from build123d import *

# Parameters (mm, degrees)
F0_W     = 81.2149718404
F0_H     = 45.3068669885
F1_DEPTH = 50.8
F2_R     = 7.5673646555
F2_R_2   = 8.1937983632
F3_DEPTH = 25.4
F5_DEPTH = 25.4
F7_DEPTH = 25.4


with BuildPart() as f1:
    # F0 (on Top) → F1 (new body)
    with BuildSketch(Plane.XY):
        with Locations((15.9056037664, 3.0124252662)):
            Rectangle(F0_W, F0_H)
    extrude(amount=F1_DEPTH)

    # F2 (on face) → F3 (cut)
    with BuildSketch(Plane.XY.offset(50.8)):
        with Locations((-12.4111901969, 4.940376617)):
            Circle(F2_R)
        with Locations((42.7764281631, 4.4583887793)):
            Circle(F2_R_2)
    extrude(amount=-F3_DEPTH, mode=Mode.SUBTRACT)

    # F4 (on face) → F5 (cut)
    with BuildSketch(Plane.XZ.offset(19.6410082281)):
        with BuildLine():
            Line((34.1006480157, 50.8), (0, 50.8))
            ThreePointArc((0, 50.8), (17.0503240079, 39.4000553567), (34.1006480157, 50.8))
        make_face()
    extrude(amount=-F5_DEPTH, mode=Mode.SUBTRACT)

    # F6 (on face) → F7 (cut)
    with BuildSketch(Plane.XZ.offset(-5.7589917719)):
        with BuildLine():
            Line((34.1006480157, 50.8), (0, 50.8))
            ThreePointArc((0, 50.8), (17.0503240079, 39.4000553567), (34.1006480157, 50.8))
        make_face()
    extrude(amount=-F7_DEPTH, mode=Mode.SUBTRACT)


solid = f1.part
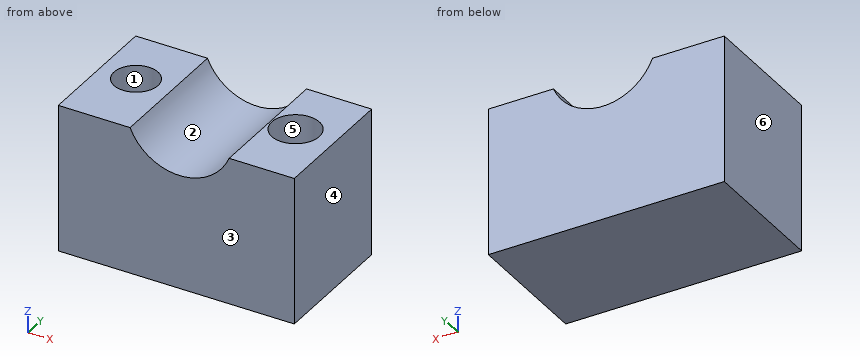
Input: part model. Units: mm. Frame: model coordinates. Face numbers are marked on the shaded views. A direction names the side the tool comes from. Coordinates: 2 decimals unless noted, no trailing zeros. Loops run counter-clockwise (first coordinate to the right, second up) from the corner with the lowest first, then second, coordinate; pieces in that order, holes last.
Q1. Draft query along X for the marked faces 1, 2, 3 and 4. Return one class per face: +X half, -X half, draft (parallel to the pull), parting line (faces both ways), or undercut.
Q2. Set-up query: the marked faces 5 and 6. Return all of +Z, -Z, +X, -X, +Y, -Y with unobstructed straight access to the full face (end or side cutting, diameter ignored); none if empty.
Q3. Material intervals for line 1 (X direction, y = -1, z = 37.5); line 2 (Z direction, x = 16.5, y = -12.5); line 3 (X direction, y = -8.5, z = 43.5), sorted ascending.
Q4. Contact query for a flat-ended pin moving along its axis: pin 1 (13 mm diameter, centred on x = 42.78, y = 4.46, fed in from +Z). Output: stop coordinate, or through.
Q5. Cut plane C-C (x = 41.5). Output: boundary loops of the cut face in (y, z).
Q6. Cut plane A-A (z = 41.5). Output: boundary loops of the cut face in (x, y), then the cut area to 3 significant figures.
Q7. Cut plane B-B (y = -8). Output: boundary loops of the cut face in (x, z), then the cut area to 3 significant figures.
Q8. Cut plane D-D (z = 48). Output: boundary loops of the cut face in (x, y), then the cut area to 3 significant figures.
Working result:
1. face 1: undercut
1. face 2: undercut
1. face 3: draft
1. face 4: +X half
2. face 5: +Z
2. face 6: +Z, -Z, -X, +Y, -Y
3. line 1: x = -24.7 to -17.1, -7.72 to 36.67, 48.89 to 56.51
3. line 2: z = 0 to 39.41
3. line 3: x = -24.7 to 5.45, 28.65 to 56.51
4. pin 1: stops at z = 25.4
5. outline: (-19.64, 0) - (25.67, 0) - (25.67, 50.8) - (12.55, 50.8) - (12.55, 25.4) - (-3.64, 25.4) - (-3.64, 50.8) - (-19.64, 50.8) - close
6. outline: (-24.7, -19.64) - (8.5, -19.64) - (8.5, 25.67) - (-24.7, 25.67) - close; (25.6, -19.64) - (56.51, -19.64) - (56.51, 25.67) - (25.6, 25.67) - close; hole circle Ø15.13 at (-12.41, 4.94); hole circle Ø16.39 at (42.78, 4.46)
6. area: 2,510 mm2
7. outline: (-24.7, 0) - (56.51, 0) - (56.51, 50.8) - (34.1, 50.8) arc R18.45 cw to (0, 50.8) - (-24.7, 50.8) - close
7. area: 3,840 mm2
8. outline: (-24.7, -19.64) - (1.45, -19.64) - (1.45, 25.67) - (-24.7, 25.67) - close; (32.65, -19.64) - (56.51, -19.64) - (56.51, 25.67) - (32.65, 25.67) - close; hole circle Ø15.13 at (-12.41, 4.94); hole circle Ø16.39 at (42.78, 4.46)
8. area: 1,880 mm2
